Verification items for the finished model (mm, model axes). A direction names the side the tool comes from. Coordinates: 2 decimals unless noted, no trailing zeros. Order: outer loops, then holes, each group sorted by start corner. A loop starts at its lowest first (then second) coordinate and runs counter-clockwise, first axis right, second up. Notation, with made-up numbers: M 43.5,81 L 82.5,81 A15 ccw 82.5,95 Z; hole C 5.25,-14 d4. An arc over 180 degrees is marked long. Return JSON: item names as keys, results as strings. Group by question number.
1. Section check D-D, the plane z = -1. Record the cut outline in (x, y), plus the area to 3 significant figures.
2. Mould release check, pull along Y, two halves, no side actions. Record for faces 1 (the flat face through (-41, 0, -11.35)), 2 (the flat face through (-38, -18, 0)), 3 (the cylindrical face through (-38.389, 12.926, -13.762)): +Y half, -Y half, draft (parallel to the pull), parting line (faces both ways), or undercut.
3. Section check C-C, the plane y = -7. Record the cut outline in (x, z).
4. Section check A-A, the plane y = 14. Record the cut outline in (x, z), plus the area to 3 significant figures.
5. Gauge pin test, flat ends, axial feed: pin 1 (2.5 mm diameter, centred on x = -40.5, y = -4, fed in from -Z); pin 2 (2 mm diameter, centred on x = -42.5, z = -2.5, fed in from -Y); pin 3 (2.5 mm diameter, centred on y = -14, z = -14, fed in from -X); pin 4 (2.5 mm diameter, centred on y = -14, z = 14, fed in from +X). Record the tip position at first contact, or that the pin passes through.
6. Material ranges on line 1 along Y through (x, z) = (-38.85, 14); line 2 along Z through (x, y) = (-40.75, 4); line 3 along X through (y, z) = (-1, -16), recorded low to high.
7. Set-up check for faces 4 (the flat face through (-43.8, 0, 0)), 5 (the flat face through (-41, -12.8, 0)), 6 (the flat face through (-41, 0, 11.35)), 7 (the flat face through (-41, 12.8, 0)): record each of +Z, -Z, +X, -X, +Y, -Y from which the full face is reachable in a straight line by a thin tool's end or side.
```python
from build123d import *

# Parameters (mm, degrees)
PLATE_START     = -37.6
PLATE_SKETCH_W  = 36
PLATE_SKETCH_H  = 36
PLATE_SKETCH_R  = 1.1
PLATE_DEPTH     = 1.6
BNO085_START    = -39.2
BNO085_SKETCH_W = 22.7
BNO085_SKETCH_H = 25.6
BNO085_DEPTH    = 4.6


with BuildPart() as part:
    # Plate Sketch → Plate (new body)
    with BuildSketch(Plane(origin=(0, 0, 0), x_dir=(0, 0, -1), z_dir=(1, 0, 0)).offset(PLATE_START)):
        Rectangle(PLATE_SKETCH_W, PLATE_SKETCH_H)
        with Locations((14, -14)):
            Circle(PLATE_SKETCH_R, mode=Mode.SUBTRACT)
        with Locations((-14, -14)):
            Circle(PLATE_SKETCH_R, mode=Mode.SUBTRACT)
        with Locations((14, 14)):
            Circle(PLATE_SKETCH_R, mode=Mode.SUBTRACT)
        with Locations((-14, 14)):
            Circle(PLATE_SKETCH_R, mode=Mode.SUBTRACT)
    extrude(amount=-PLATE_DEPTH)

    # BNO085 Sketch → BNO085 (add)
    with BuildSketch(Plane(origin=(0, 0, 0), x_dir=(0, 0, -1), z_dir=(1, 0, 0)).offset(BNO085_START)):
        Rectangle(BNO085_SKETCH_W, BNO085_SKETCH_H)
    extrude(amount=-BNO085_DEPTH)


solid = part.part
```
Answers follow:
{
 "1": {"outline": "M -43.8,-12.8 L -39.2,-12.8 L -39.2,-18 L -37.6,-18 L -37.6,18 L -39.2,18 L -39.2,12.8 L -43.8,12.8 Z", "area": "175 mm^2"},
 "2": {"face 1": "draft", "face 2": "-Y half", "face 3": "undercut"},
 "3": {"outline": "M -43.8,-11.35 L -39.2,-11.35 L -39.2,-18 L -37.6,-18 L -37.6,18 L -39.2,18 L -39.2,11.35 L -43.8,11.35 Z"},
 "4": {"outline": "M -39.2,-18 L -37.6,-18 L -37.6,-15.1 L -39.2,-15.1 Z; M -39.2,-12.9 L -37.6,-12.9 L -37.6,12.9 L -39.2,12.9 Z; M -39.2,15.1 L -37.6,15.1 L -37.6,18 L -39.2,18 Z", "area": "50.6 mm^2"},
 "5": {"pin 1": "z = -11.35", "pin 2": "y = -12.8", "pin 3": "x = -39.2", "pin 4": "x = -37.6"},
 "6": {"line 1": "-18 to -15.1, -12.9 to 12.9, 15.1 to 18", "line 2": "-11.35 to 11.35", "line 3": "-39.2 to -37.6"},
 "7": {"face 4": "+Z, -Z, -X, +Y, -Y", "face 5": "+Z, -Z, -X, -Y", "face 6": "+Z, -X, +Y, -Y", "face 7": "+Z, -Z, -X, +Y"}
}
